Autodesk Inventor part; units mm, degrees
ref_plane "YZ Plane" through (0, 0, 0) normal (1, 0, 0) x (0, 1, 0)
ref_plane "XZ Plane" through (0, 0, 0) normal (0, 1, 0) x (-1, 0, 0)
ref_plane "XY Plane" through (0, 0, 0) normal (0, 0, 1) x (1, 0, 0)
sketch "Sketch2" plane through (0, 0, 0) normal (0, 0, 1) x (1, 0, 0)
  line L0 (40, -40) -> (-40, -40)
  line L1 (-40, -40) -> (-40, 40)
  line L2 (-40, 40) -> (40, 40)
  line L3 (40, 40) -> (40, -40)
  line L4 (-56, 0) -> (56, 0) construction
  line L5 (0, 56) -> (0, -56) construction
  line L6 (-30, 33.25) -> (-30, 11.75) construction
  line L7 (-33.25, 30) -> (-33.25, 15)
  line L8 (-26.75, 15) -> (-26.75, 30)
  arc A0 (-26.75, 30) -> (-33.25, 30) centre (-30, 30) ccw
  arc A1 (-33.25, 15) -> (-26.75, 15) centre (-30, 15) ccw
  line L9 (-26.75, -30) -> (-26.75, -15)
  arc A2 (-26.75, -15) -> (-33.25, -15) centre (-30, -15) ccw
  line L10 (-33.25, -15) -> (-33.25, -30)
  arc A3 (-33.25, -30) -> (-26.75, -30) centre (-30, -30) ccw
  line L11 (33.25, 15) -> (33.25, 30)
  arc A4 (33.25, 30) -> (26.75, 30) centre (30, 30) ccw
  line L12 (26.75, 30) -> (26.75, 15)
  arc A5 (26.75, 15) -> (33.25, 15) centre (30, 15) ccw
  line L13 (33.25, -30) -> (33.25, -15)
  arc A6 (33.25, -15) -> (26.75, -15) centre (30, -15) ccw
  line L14 (26.75, -15) -> (26.75, -30)
  arc A7 (26.75, -30) -> (33.25, -30) centre (30, -30) ccw
  point P0 (0, 0)
  point P1 (0, 0)
  point P2 (0, 0)
  point P3 (-30, 22.5)
  dimension "d10" = 80
  dimension "d11" = 80
  dimension "d12" = 40
  dimension "d13" = 40
  dimension "d14" = 6.5
  dimension "d15" = 10
  dimension "d16" = 10
  dimension "d17" = 15
  dimension "d20" = 45
  dimension "d23" = 60
  dimension "d26" = 6.75
extrude "Extrusion1" add sketch "Sketch2" along normal blind 4
sketch "Sketch3" plane through (0, 0, 0) normal (1, 0, 0) x (0, 1, 0)
  line L0 (33.25, 4) -> (33.25, 0) construction
  line L1 (11.75, 4) -> (11.75, 0) construction
  line L2 (30, 0) -> (15, 0) construction
  line L3 (15, 0) -> (15, 4) construction
  line L4 (30, 4) -> (15, 4) construction
  line L5 (30, 0) -> (30, 4) construction
  line L6 (-15, 0) -> (-30, 0) construction
  line L7 (-30, 0) -> (-30, 4) construction
  line L8 (-15, 4) -> (-30, 4) construction
  line L9 (-15, 0) -> (-15, 4) construction
  line L10 (40, 0) -> (-40, 0) construction
  line L11 (-40, 0) -> (-40, 4) construction
  line L12 (40, 4) -> (-40, 4) construction
  line L13 (40, 0) -> (40, 4) construction
  line L14 (40, 4) -> (40, 84)
  line L15 (40, 84) -> (27.128, 84)
  line L16 (27.128, 84) -> (-40, 4)
  line L17 (-33.25, 4) -> (-33.25, 0) construction
  line L18 (-11.75, 4) -> (-11.75, 0) construction
  line L19 (-30, 8.0014) -> (-15, 8.0014)
  line L20 (15, 8) -> (30, 8)
  line L21 (-15, 8.0014) -> (-15, 4)
  line L22 (-30, 8.0014) -> (-30, 4)
  line L23 (30, 8) -> (30, 4)
  line L24 (15, 8) -> (15, 4)
  line L25 (30, 4) -> (40, 4)
  line L26 (15, 4) -> (-15, 4)
  line L27 (-30, 4) -> (-40, 4)
  point P0 (0, 0)
  dimension "d29" = 80
  dimension "d30" = 4
  dimension "d32" = 130
  dimension "d34" = 4.0014
extrude "Extrusion2" add sketch "Sketch3" along normal mid plane 4
fillet "Fillet1" radius 2 6 edges at (-2, 0, 4) (-2, 35, 4) (-2, -35, 4) (2, 0, 4) (2, 35, 4) (2, -35, 4)
fillet "Fillet2" radius 2 2 edges at (0, 27.128, 84) (0, 40, 84)
sketch "Sketch4" plane through (2, 0, 0) normal (1, 0, 0) x (0, 0, -1)
  arc A0 (-82, 40) -> (-84, 38) centre (-82, 38) ccw construction
  line L0 (-84, 38) -> (-84, 28.0606) construction
  arc A1 (-84, 28.0606) -> (-83.2856, 26.5285) centre (-82, 28.0606) ccw construction
  line L1 (-83.2856, 26.5285) -> (-6, -38.3218) construction
  line L2 (-6, -30) -> (-6, -38.3218) construction
  line L3 (-6, -30) -> (-8.0014, -30) construction
  line L4 (-8.0014, -30) -> (-8.0014, -15) construction
  line L5 (-8.0014, -15) -> (-6, -15) construction
  line L6 (-6, 15) -> (-6, -15) construction
  line L7 (-6, 15) -> (-8, 15) construction
  line L8 (-8, 15) -> (-8, 30) construction
  line L9 (-8, 30) -> (-6, 30) construction
  line L10 (-6, 40) -> (-6, 30) construction
  line L11 (-6, 40) -> (-82, 40) construction
  point P0 (0, 0)
  point P1 (-72, 30)
  dimension "d39" = 12
  dimension "d40" = 10
hole "Hole1" at (2, 30, 72) direction (-1, 0, 0) diameter 9 depth 10
properties part number "P045_SupportUniversel"
Work out the finished part from the listing and answer in its coordinate system (mm). A direction names the side the tool comes from. Round coordinates to 2 decimals unless told otherwise and drop trailing zeros. Write each loop counter-clockwise with the first axis right and the second up, starting at its lowest first coordinate (ties: lowest second). Pieces come first, ordered by that corner, then holes.
1) Flat-ended cylindrical pins translate along their axes: P1, Ø5, axis at x = 2.5, y = -14, coming from the +Z side; P2, Ø1.5, axis at y = 22, z = 26, coming from the -X side; P3, Ø3, axis at x = 1.5, z = 7, coming from the -Y side. Find the tip coordinate at first contact, or state that the pin passes through.
2) A cutting plane is placed at D-D on x = -30.5. Determine the outline of the cut face in (y, z).
3) A cutting plane is placed at B-B on z = 72. Determine the outline of the cut face in (x, y).
4) Which of the six approach directions +Z, -Z, +X, -X, +Y, -Y give full straight-line access (tool end or side, diameter ignored) to faces 4 (the face through (0, 15, 6)), 5 (the face through (-26.75, -23, 2)), 6 (the face through (2, 9, 37))?
5) A cutting plane is placed at A-A on x = 30. Determine the outline of the cut face in (y, z).
6) A cutting plane is placed at C-C on y = -0.5. Determine the outline of the cut face in (x, z).
7) Consider probe 1 along Z at (x, y) = (23, -15); probe 2 along X at (y, z) = (-11.5, 6); probe 3 along Y at (x, z) = (0, 73). Determine where each line is inside the solid, lowest interval first.
8) Determine the mould class of faces 1 (the face through (0, 33, 84)), 2 (the face through (0, -23, 8.001)), 3 (the face through (29.93, 33.25, 1.97)) for opening direction Z: pulls with the +Z half, pulls with the -Z half, needs draft (parallel to the pull), parting line crosses it, or undercut.
Entries:
1. P1: stops at z = 37.9
1. P2: stops at x = -2
1. P3: stops at y = -38.74
2. outline: (-40, 0) - (-33.21, 0) - (-33.21, 4) - (-40, 4) - close; (-11.79, 0) - (11.79, 0) - (11.79, 4) - (-11.79, 4) - close; (33.21, 0) - (40, 0) - (40, 4) - (33.21, 4) - close
3. outline: (-2, 17.06) - (2, 17.06) - (2, 25.5) - (-2, 25.5) - close; (-2, 34.5) - (2, 34.5) - (2, 40) - (-2, 40) - close
4. face 4: +X, -X
4. face 5: +Z, -Z
4. face 6: +Z, +X, +Y, -Y
5. outline: (-40, 0) - (-33.25, 0) - (-33.25, 4) - (-40, 4) - close; (-11.75, 0) - (11.75, 0) - (11.75, 4) - (-11.75, 4) - close; (33.25, 0) - (40, 0) - (40, 4) - (33.25, 4) - close
6. outline: (-40, 0) - (40, 0) - (40, 4) - (4, 4) arc R2 cw to (2, 6) - (2, 51.07) - (-2, 51.07) - (-2, 6) arc R2 cw to (-4, 4) - (-40, 4) - close
7. probe 1: z = 0 to 4
7. probe 2: x = -2 to 2
7. probe 3: y = 17.9 to 25.61, 34.39 to 40
8. face 1: pulls with the +Z half
8. face 2: undercut
8. face 3: needs draft
